Design review of the part built by this model. Coordinates are the model's own, in mm. A direction names the side the tool comes from. Give positions to 0.01 mm unless a question says otherwise; leave off trailing zeros. Order: outer loops, then holes, each group sorted by start corner. A loop starts at its lowest first (then second) coordinate and runs counter-clockwise, first axis right, second up. Notation, with made-up numbers: (-18, 67) -> (-7, 67) arc R5 ccw to (-7, 75) -> close; hole circle Ø6 at (43, -30). An arc over 180 degrees is marked (long way). One line per item, written item: value.
from build123d import *

# Parameters (mm, degrees)
F1_DEPTH = 15
F3_DEPTH = 3
F4_F1_R  = 0.5
F4_F2_R  = 0.5
F4_F3_R  = 0.5
F4_F4_R  = 0.5


with BuildPart() as f1:
    # F0 (on Top) → F1 (new body)
    with BuildSketch(Plane.XY):
        with BuildLine():
            Line((35.5372718227, 19.9606023237), (-30.4627281773, 19.9606023237))
            ThreePointArc((-30.4627281773, 19.9606023237), (-30.8162815679, 19.8141557143), (-30.9627281773, 19.4606023237))
            Line((-30.9627281773, 19.4606023237), (-30.9627281773, -36.5393976763))
            ThreePointArc((-30.9627281773, -36.5393976763), (-30.8162815679, -36.8929510669), (-30.4627281773, -37.0393976763))
            Line((-30.4627281773, -37.0393976763), (35.5372718227, -37.0393976763))
            ThreePointArc((35.5372718227, -37.0393976763), (35.8908252133, -36.8929510669), (36.0372718227, -36.5393976763))
            Line((36.0372718227, -36.5393976763), (36.0372718227, 19.4606023237))
            ThreePointArc((36.0372718227, 19.4606023237), (35.8908252133, 19.8141557143), (35.5372718227, 19.9606023237))
        make_face()
        with BuildLine():
            ThreePointArc((-27.9627281773, 16.4606023237), (-27.8162815679, 16.8141557143), (-27.4627281773, 16.9606023237))
            Line((-27.4627281773, 16.9606023237), (32.5372718227, 16.9606023237))
            ThreePointArc((32.5372718227, 16.9606023237), (32.8908252133, 16.8141557143), (33.0372718227, 16.4606023237))
            Line((33.0372718227, 16.4606023237), (33.0372718227, -33.5393976763))
            ThreePointArc((33.0372718227, -33.5393976763), (32.8908252133, -33.8929510669), (32.5372718227, -34.0393976763))
            Line((32.5372718227, -34.0393976763), (-27.4627281773, -34.0393976763))
            ThreePointArc((-27.4627281773, -34.0393976763), (-27.8162815679, -33.8929510669), (-27.9627281773, -33.5393976763))
            Line((-27.9627281773, -33.5393976763), (-27.9627281773, 16.4606023237))
        make_face(mode=Mode.SUBTRACT)
    extrude(amount=F1_DEPTH)

    # F2 (on face) → F3 (join)
    with BuildSketch(Plane.XY.offset(15)):
        with BuildLine():
            Line((-15.9627281773, -34.0393976763), (-15.9627281773, 16.9606023237))
            Line((-15.9627281773, 16.9606023237), (-27.4627281773, 16.9606023237))
            ThreePointArc((-27.4627281773, 16.9606023237), (-27.8162815679, 16.8141557143), (-27.9627281773, 16.4606023237))
            Line((-27.9627281773, 16.4606023237), (-27.9627281773, -33.5393976763))
            ThreePointArc((-27.9627281773, -33.5393976763), (-27.8162815679, -33.8929510669), (-27.4627281773, -34.0393976763))
            Line((-27.4627281773, -34.0393976763), (-15.9627281773, -34.0393976763))
        make_face()
        with BuildLine():
            ThreePointArc((-30.4627281773, 19.9606023237), (-30.8162815679, 19.8141557143), (-30.9627281773, 19.4606023237))
            Line((-30.9627281773, 19.4606023237), (-30.9627281773, -36.5393976763))
            ThreePointArc((-30.9627281773, -36.5393976763), (-30.8162815679, -36.8929510669), (-30.4627281773, -37.0393976763))
            Line((-30.4627281773, -37.0393976763), (-15.9627281773, -37.0393976763))
            Line((-15.9627281773, -37.0393976763), (-15.9627281773, -34.0393976763))
            Line((-15.9627281773, -34.0393976763), (-27.4627281773, -34.0393976763))
            ThreePointArc((-27.4627281773, -34.0393976763), (-27.8162815679, -33.8929510669), (-27.9627281773, -33.5393976763))
            Line((-27.9627281773, -33.5393976763), (-27.9627281773, 16.4606023237))
            ThreePointArc((-27.9627281773, 16.4606023237), (-27.8162815679, 16.8141557143), (-27.4627281773, 16.9606023237))
            Line((-27.4627281773, 16.9606023237), (-15.9627281773, 16.9606023237))
            Line((-15.9627281773, 16.9606023237), (-15.9627281773, 19.9606023237))
            Line((-15.9627281773, 19.9606023237), (-30.4627281773, 19.9606023237))
        make_face()
        with BuildLine():
            Line((35.5372718227, 19.9606023237), (-15.9627281773, 19.9606023237))
            Line((-15.9627281773, 19.9606023237), (-15.9627281773, 16.9606023237))
            Line((-15.9627281773, 16.9606023237), (32.5372718227, 16.9606023237))
            ThreePointArc((32.5372718227, 16.9606023237), (32.8908252133, 16.8141557143), (33.0372718227, 16.4606023237))
            Line((33.0372718227, 16.4606023237), (33.0372718227, -33.5393976763))
            ThreePointArc((33.0372718227, -33.5393976763), (32.8908252133, -33.8929510669), (32.5372718227, -34.0393976763))
            Line((32.5372718227, -34.0393976763), (-15.9627281773, -34.0393976763))
            Line((-15.9627281773, -34.0393976763), (-15.9627281773, -37.0393976763))
            Line((-15.9627281773, -37.0393976763), (35.5372718227, -37.0393976763))
            ThreePointArc((35.5372718227, -37.0393976763), (35.8908252133, -36.8929510669), (36.0372718227, -36.5393976763))
            Line((36.0372718227, -36.5393976763), (36.0372718227, 19.4606023237))
            ThreePointArc((36.0372718227, 19.4606023237), (35.8908252133, 19.8141557143), (35.5372718227, 19.9606023237))
        make_face()
    extrude(amount=F3_DEPTH)

    # F4: fillet of radius 0.5 on 7 edges, made by hand

    # F4_f1
    f4_f1_edges = [f1.edges().sort_by_distance(p)[0] for p in [
        (2.5372718227, 19.9606023237, 18),
        (36.0372718227, -8.5393976763, 18),
        (35.8908252133, -36.8929510669, 18),
        (2.5372718227, -37.0393976763, 18),
        (-30.8162815679, -36.8929510669, 18),
        (-30.9627281773, -8.5393976763, 18),
        (-30.8162815679, 19.8141557143, 18),
        (35.8908252133, 19.8141557143, 18),
    ]]
    fillet(f4_f1_edges, radius=F4_F1_R)

    # F4_f2
    f4_f2_edges = [f1.edges().sort_by_distance(p)[0] for p in [
        (-15.9627281773, -8.5393976763, 15),
    ]]
    fillet(f4_f2_edges, radius=F4_F2_R)

    # F4_f3
    f4_f3_edges = [f1.edges().sort_by_distance(p)[0] for p in [
        (-15.9627281773, -34.0393976763, 16.75),
    ]]
    fillet(f4_f3_edges, radius=F4_F3_R)

    # F4_f4
    f4_f4_edges = [f1.edges().sort_by_distance(p)[0] for p in [
        (-15.9627281773, -8.5393976763, 18),
    ]]
    fillet(f4_f4_edges, radius=F4_F4_R)


solid = f1.part
Item 1: To check wall thickness, follow line 1 along X through (y, z) = (-10, 6); line 2 along Y through (x, z) = (12, 4.25); line 3 along X through (y, z) = (7, 16.5). State the ranges of each line that lie inside material, in increasing order. Write a range as from..to.
Returned:
line 1: -30.96..-27.96, 33.04..36.04
line 2: -37.04..-34.04, 16.96..19.96
line 3: -30.96..-15.96, 33.04..36.04
Item 2: Clearance check with a flat-ended pin moving along its axis: P1, Ø5.5, axis at x = -20, y = -14.5, coming from the -Z side. State where the tip first meets the part, or that it passes through.
Returned:
P1: z = 15
Item 3: Add section C-C on y = 2.5. Give the boundary of the cut face in (x, z).
Returned:
outline: (-30.96, 0) -> (-27.96, 0) -> (-27.96, 14.5) arc R0.5 cw to (-27.46, 15) -> (-16.46, 15) arc R0.5 ccw to (-15.96, 15.5) -> (-15.96, 17.5) arc R0.5 ccw to (-16.46, 18) -> (-30.46, 18) arc R0.5 ccw to (-30.96, 17.5) -> close; (33.04, 0) -> (36.04, 0) -> (36.04, 17.5) arc R0.5 ccw to (35.54, 18) -> (33.54, 18) arc R0.5 ccw to (33.04, 17.5) -> close
Item 4: Machinability: for faces 1 (the flat face through (2, -37.039, 9)), 2 (the flat face through (-15.963, -9, 16)), 3 (the flat face through (2, 16.961, 9)), which of the approach directions +Z, -Z, +X, -X, +Y, -Y give a long, thin tool a straight path to every point of the face, cutting with its end or side? Answer none if there is none.
Returned:
face 1: +Z, -Z, +X, -X, -Y
face 2: +Z, -Z
face 3: -Z
Item 5: Add section B-B on x = -0.5. Give the boundary of the cut face in (y, z).
Returned:
outline: (-37.04, 0) -> (-34.04, 0) -> (-34.04, 17.5) arc R0.5 ccw to (-34.54, 18) -> (-36.54, 18) arc R0.5 ccw to (-37.04, 17.5) -> close; (16.96, 0) -> (19.96, 0) -> (19.96, 17.5) arc R0.5 ccw to (19.46, 18) -> (17.46, 18) arc R0.5 ccw to (16.96, 17.5) -> close
Item 6: Add section D-D on x = -20. Give the boundary of the cut face in (y, z), plus the area to 3 significant figures.
Returned:
outline: (-37.04, 0) -> (-34.04, 0) -> (-34.04, 14.5) arc R0.5 cw to (-33.54, 15) -> (16.46, 15) arc R0.5 cw to (16.96, 14.5) -> (16.96, 0) -> (19.96, 0) -> (19.96, 17.5) arc R0.5 ccw to (19.46, 18) -> (-36.54, 18) arc R0.5 ccw to (-37.04, 17.5) -> close
area: 261 mm²
Item 7: Draft analysis for pull direction Y (two halves, no side actions). For faces 4 (the flat face through (33.037, -8, 9)), 5 (the flat face through (3, 19.961, 9)), 6 (the flat face through (3, -34.039, 9)), 7 (the flat face through (-30.963, -8, 9)), state which applies: pulls with the +Y half, pulls with the -Y half, needs draft (parallel to the pull), parting line crosses it, or undercut.
Returned:
face 4: undercut
face 5: pulls with the +Y half
face 6: undercut
face 7: needs draft
Item 8: Add section A-A on z = 11.25. Give the boundary of the cut face in (x, y), plus the area to 3 significant figures.
Returned:
outline: (-30.96, -36.54) arc R0.5 ccw to (-30.46, -37.04) -> (35.54, -37.04) arc R0.5 ccw to (36.04, -36.54) -> (36.04, 19.46) arc R0.5 ccw to (35.54, 19.96) -> (-30.46, 19.96) arc R0.5 ccw to (-30.96, 19.46) -> close; hole (-27.96, -33.54) arc R0.5 ccw to (-27.46, -34.04) -> (32.54, -34.04) arc R0.5 ccw to (33.04, -33.54) -> (33.04, 16.46) arc R0.5 ccw to (32.54, 16.96) -> (-27.46, 16.96) arc R0.5 ccw to (-27.96, 16.46) -> close
area: 708 mm²
